Read the model definition and answer for the solid it produces. Units are mm, in the model's axes. A direction names the side the tool comes from. Coordinates: 2 decimals unless noted, no trailing zeros. Loops run counter-clockwise (first coordinate to the right, second up) from the corner with the lowest first, then second, coordinate; pieces in that order, holes last. Notation, with made-up numbers: M -22,89 L 28,89 A6 cw 28,93 Z; hole C -34,-25.5 d2. An arc over 180 degrees is marked long. Put each result on its own line as item: value.
from build123d import *

# Parameters (mm, degrees)
SKETCH2_W           = 50
SKETCH2_H           = 20
BOSS_EXTRUDE1_DEPTH = 10
SKETCH3_R           = 1.3
SKETCH3_R_2         = 1.35
SKETCH3_R_3         = 1.4
SKETCH3_R_4         = 1.45
SKETCH3_R_5         = 1.5
SKETCH3_R_6         = 1.55
SKETCH3_R_7         = 1.6
SKETCH3_R_8         = 1.65
CUT_EXTRUDE1_DEPTH  = 29.722813233


with BuildPart() as part:
    # Sketch2 → Boss-Extrude1 (new body)
    with BuildSketch(Plane(origin=(0, 0, 0), x_dir=(1, 0, 0), z_dir=(0, 1, 0))):
        Rectangle(SKETCH2_W, SKETCH2_H)
    extrude(amount=BOSS_EXTRUDE1_DEPTH)

    # Sketch3 → Cut-Extrude1 (cut, through all)
    with BuildSketch(Plane(origin=(0, 10, 0), x_dir=(1, 0, 0), z_dir=(0, 1, 0))):
        with Locations(Location((-19.685722489, 6.222302146, 0), (0, 0, 270))):
            Circle(SKETCH3_R)
        with Locations(Location((-14.685722489, 6.222302146, 0), (0, 0, 270))):
            Circle(SKETCH3_R_2)
        with Locations(Location((-9.685722489, 6.222302146, 0), (0, 0, 270))):
            Circle(SKETCH3_R_3)
        with Locations(Location((-4.685722489, 6.222302146, 0), (0, 0, 270))):
            Circle(SKETCH3_R_4)
        with Locations(Location((0.314277511, 6.222302146, 0), (0, 0, 270))):
            Circle(SKETCH3_R_5)
        with Locations(Location((5.314277511, 6.222302146, 0), (0, 0, 270))):
            Circle(SKETCH3_R_6)
        with Locations(Location((10.314277511, 6.222302146, 0), (0, 0, 270))):
            Circle(SKETCH3_R_7)
        with Locations(Location((15.314277511, 6.222302146, 0), (0, 0, 270))):
            Circle(SKETCH3_R_8)
        with BuildLine():
            Line((6.65, -10), (3.35, -10))
            Line((3.35, -10), (3.35, -6.2))
            Line((3.35, -6.2), (2.25, -6.2))
            ThreePointArc((2.25, -6.2), (2.073223305, -6.126776695), (2, -5.95))
            Line((2, -5.95), (2, -2.25))
            ThreePointArc((2, -2.25), (2.073223305, -2.073223305), (2.25, -2))
            Line((2.25, -2), (3.35, -2))
            Line((3.35, -2), (3.35, 0.5))
            Line((3.35, 0.5), (6.65, 0.5))
            Line((6.65, 0.5), (6.65, -2))
            Line((6.65, -2), (7.75, -2))
            ThreePointArc((7.75, -2), (7.926776695, -2.073223305), (8, -2.25))
            Line((8, -2.25), (8, -5.95))
            ThreePointArc((8, -5.95), (7.926776695, -6.126776695), (7.75, -6.2))
            Line((7.75, -6.2), (6.65, -6.2))
            Line((6.65, -6.2), (6.65, -10))
        make_face()
        with BuildLine():
            Line((15.25, 0.5), (18.75, 0.5))
            Line((18.75, 0.5), (18.75, -2))
            Line((18.75, -2), (19.85, -2))
            ThreePointArc((19.85, -2), (20.026776695, -2.073223305), (20.1, -2.25))
            Line((20.1, -2.25), (20.1, -5.95))
            ThreePointArc((20.1, -5.95), (20.026776695, -6.126776695), (19.85, -6.2))
            Line((19.85, -6.2), (18.75, -6.2))
            Line((18.75, -6.2), (18.75, -10))
            Line((18.75, -10), (15.25, -10))
            Line((15.25, -10), (15.25, -6.2))
            Line((15.25, -6.2), (14.15, -6.2))
            ThreePointArc((14.15, -6.2), (13.973223305, -6.126776695), (13.9, -5.95))
            Line((13.9, -5.95), (13.9, -2.25))
            ThreePointArc((13.9, -2.25), (13.973223305, -2.073223305), (14.15, -2))
            Line((14.15, -2), (15.25, -2))
            Line((15.25, -2), (15.25, 0.5))
        make_face()
        with BuildLine():
            Line((-8.55, 0.5), (-5.45, 0.5))
            Line((-5.45, 0.5), (-5.45, -2))
            Line((-5.45, -2), (-4.35, -2))
            ThreePointArc((-4.35, -2), (-4.173223305, -2.073223305), (-4.1, -2.25))
            Line((-4.1, -2.25), (-4.1, -5.95))
            ThreePointArc((-4.1, -5.95), (-4.173223305, -6.126776695), (-4.35, -6.2))
            Line((-4.35, -6.2), (-5.45, -6.2))
            Line((-5.45, -6.2), (-5.45, -10))
            Line((-5.45, -10), (-8.55, -10))
            Line((-8.55, -10), (-8.55, -6.2))
            Line((-8.55, -6.2), (-9.65, -6.2))
            ThreePointArc((-9.65, -6.2), (-9.826776695, -6.126776695), (-9.9, -5.95))
            Line((-9.9, -5.95), (-9.9, -2.25))
            ThreePointArc((-9.9, -2.25), (-9.826776695, -2.073223305), (-9.65, -2))
            Line((-9.65, -2), (-8.55, -2))
            Line((-8.55, -2), (-8.55, 0.5))
        make_face()
        with BuildLine():
            Line((-20.55, 0.5), (-17.45, 0.5))
            Line((-17.45, 0.5), (-17.45, -3))
            Line((-17.45, -3), (-16.25, -3))
            ThreePointArc((-16.25, -3), (-16.073223305, -3.073223305), (-16, -3.25))
            Line((-16, -3.25), (-16, -5.75))
            ThreePointArc((-16, -5.75), (-16.073223305, -5.926776695), (-16.25, -6))
            Line((-16.25, -6), (-17.45, -6))
            Line((-17.45, -6), (-17.45, -10))
            Line((-17.45, -10), (-20.55, -10))
            Line((-20.55, -10), (-20.55, -6))
            Line((-20.55, -6), (-21.75, -6))
            ThreePointArc((-21.75, -6), (-21.926776695, -5.926776695), (-22, -5.75))
            Line((-22, -5.75), (-22, -3.25))
            ThreePointArc((-22, -3.25), (-21.926776695, -3.073223305), (-21.75, -3))
            Line((-21.75, -3), (-20.55, -3))
            Line((-20.55, -3), (-20.55, 0.5))
        make_face()
    extrude(amount=-CUT_EXTRUDE1_DEPTH, mode=Mode.SUBTRACT)


solid = part.part
1) Straight lines are drawn through the part: line 1 (X direction, y = 5, z = 7); line 2 (X direction, y = 4.5, z = 5); line 3 (Z direction, x = 3, y = 7.75). For each, find the intervals that lie inside material, in ascending order. Write a range as [from, to].
Answer list:
line 1: x = [-25, -20.55], [-17.45, -8.55], [-5.45, 3.35], [6.65, 15.25], [18.75, 25]
line 2: x = [-25, -22], [-16, -9.9], [-4.1, 2], [8, 13.9], [20.1, 25]
line 3: z = [-10, 2], [6.2, 10]
2) Find section A-A, the plane z = 0. Write down the section's boundary in (x, y).
Answer list:
outline: M -25,0 L -20.55,0 L -20.55,10 L -25,10 Z; M -17.45,0 L -8.55,0 L -8.55,10 L -17.45,10 Z; M -5.45,0 L 3.35,0 L 3.35,10 L -5.45,10 Z; M 6.65,0 L 15.25,0 L 15.25,10 L 6.65,10 Z; M 18.75,0 L 25,0 L 25,10 L 18.75,10 Z
3) Determine the mould class of faces 1 (the flat face through (-5.45, 5, 8)), 2 (the flat face through (-25, 5, 0)), 3 (the flat face through (-1, 5, 10)) for opening direction X: released by +X, released by -X, zero draft, split by the parting line, or undercut.
Answer list:
face 1: undercut
face 2: released by -X
face 3: zero draft
4) Find section C-C, the plane y = 7.5. Count the separate pieces of the cut face and the enclosed holes in it, plus the area to 3 significant figures.
Answer list:
separate pieces: 1
enclosed holes: 8
area: 766 mm^2
5) Find section D-D, the plane x = -7. Write down the section's boundary in (y, z).
Answer list:
outline: M 0,-10 L 10,-10 L 10,-0.5 L 0,-0.5 Z
6) Find section B-B, the plane x = -19. Write down the section's boundary in (y, z).
Answer list:
outline: M 0,-10 L 10,-10 L 10,-7.33 L 0,-7.33 Z; M 0,-5.12 L 10,-5.12 L 10,-0.5 L 0,-0.5 Z
7) Which of the six approach directions +Z, -Z, +X, -X, +Y, -Y give full straight-line access (tool end or side, diameter ignored) to faces 4 (the flat face through (18.75, 5, 8)), 5 (the flat face through (15, 5, 2))?
Answer list:
face 4: +Z, +Y, -Y
face 5: +Y, -Y
